```python
from build123d import *

# Parameters (mm, degrees)
SKETCH1_R       = 1
SKETCH1_R_2     = 3.5
SKETCH1_R_3     = 1.5
SKETCH1_W       = 58.004829366
SKETCH1_H       = 74
SKETCH1_W_2     = 12.5
SKETCH1_H_2     = 23.5
EXTRUDE_1_DEPTH = 3


with BuildPart() as part:
    # Sketch1 → Бобышка-Вытянуть1 (new body)
    with BuildSketch(Plane.XY):
        with BuildLine():
            Line((-24.498196466, 18.686253871), (-28.812938034, 21.763271713))
            ThreePointArc((-28.812938034, 21.763271713), (-34.033313652, 22.967935089), (-38.576502294, 20.128397731))
            Line((-38.576502294, 20.128397731), (-42.0602267, 15.24335277))
            ThreePointArc((-42.0602267, 15.24335277), (-43.264890076, 10.022977152), (-40.425352718, 5.47978851))
            Line((-40.425352718, 5.47978851), (-36.440527218, 2.638047245))
            ThreePointArc((-36.440527218, 2.638047245), (-34.281914219, 0.144259766), (-33.504872357, -3.061171876))
            Line((-33.504872357, -3.061171876), (-33.504872357, -48.061171876))
            ThreePointArc((-33.504872357, -48.061171876), (-34.969338451, -51.596705782), (-38.504872357, -53.061171876))
            Line((-38.504872357, -53.061171876), (-42.504872357, -53.061171876))
            ThreePointArc((-42.504872357, -53.061171876), (-47.454619825, -55.111424408), (-49.504872357, -60.061171876))
            Line((-49.504872357, -60.061171876), (-49.500334917, -60.235639257))
            Line((-49.500334917, -60.235639257), (-49.500334917, -66.108369799))
            Line((-49.500334917, -66.108369799), (-49.504872357, -66.28283718))
            ThreePointArc((-49.504872357, -66.28283718), (-47.454619825, -71.232584649), (-42.504872357, -73.28283718))
            Line((-42.504872357, -73.28283718), (-38.504872357, -73.28283718))
            ThreePointArc((-38.504872357, -73.28283718), (-34.969338451, -74.747303275), (-33.504872357, -78.28283718))
            Line((-33.504872357, -78.28283718), (-33.504872357, -123.28283718))
            ThreePointArc((-33.504872357, -123.28283718), (-34.281914219, -126.488268823), (-36.440527218, -128.982056301))
            Line((-36.440527218, -128.982056301), (-40.425352718, -131.823797566))
            ThreePointArc((-40.425352718, -131.823797566), (-43.264890076, -136.366986209), (-42.0602267, -141.587361827))
            Line((-42.0602267, -141.587361827), (-38.576502294, -146.472406787))
            ThreePointArc((-38.576502294, -146.472406787), (-34.033313652, -149.311944145), (-28.812938034, -148.107280769))
            Line((-28.812938034, -148.107280769), (-24.498196466, -145.030262927))
            ThreePointArc((-24.498196466, -145.030262927), (-21.740151192, -143.647892601), (-18.691989124, -143.172004528))
            Line((-18.691989124, -143.172004528), (46.687073776, -143.172004528))
            ThreePointArc((46.687073776, -143.172004528), (49.735235844, -143.647892601), (52.493281118, -145.030262927))
            Line((52.493281118, -145.030262927), (56.808022686, -148.107280769))
            ThreePointArc((56.808022686, -148.107280769), (62.028398304, -149.311944145), (66.571586947, -146.472406787))
            Line((66.571586947, -146.472406787), (70.055311352, -141.587361827))
            ThreePointArc((70.055311352, -141.587361827), (71.259974728, -136.366986209), (68.42043737, -131.823797566))
            Line((68.42043737, -131.823797566), (64.43561187, -128.982056301))
            ThreePointArc((64.43561187, -128.982056301), (62.276998871, -126.488268823), (61.499957009, -123.28283718))
            Line((61.499957009, -123.28283718), (61.499957009, -78.28283718))
            ThreePointArc((61.499957009, -78.28283718), (62.964423103, -74.747303275), (66.499957009, -73.28283718))
            Line((66.499957009, -73.28283718), (70.499957009, -73.28283718))
            ThreePointArc((70.499957009, -73.28283718), (75.449704478, -71.232584649), (77.499957009, -66.28283718))
            Line((77.499957009, -66.28283718), (77.495419569, -66.108369799))
            Line((77.495419569, -66.108369799), (77.495419569, -60.235639257))
            Line((77.495419569, -60.235639257), (77.499957009, -60.061171876))
            ThreePointArc((77.499957009, -60.061171876), (75.449704478, -55.111424407), (70.499957009, -53.061171876))
            Line((70.499957009, -53.061171876), (66.499957009, -53.061171876))
            ThreePointArc((66.499957009, -53.061171876), (62.964423103, -51.596705782), (61.499957009, -48.061171876))
            Line((61.499957009, -48.061171876), (61.499957009, -3.061171876))
            ThreePointArc((61.499957009, -3.061171876), (62.276998871, 0.144259766), (64.43561187, 2.638047245))
            Line((64.43561187, 2.638047245), (68.42043737, 5.47978851))
            ThreePointArc((68.42043737, 5.47978851), (71.259974728, 10.022977152), (70.055311352, 15.24335277))
            Line((70.055311352, 15.24335277), (66.571586947, 20.128397731))
            ThreePointArc((66.571586947, 20.128397731), (62.028398304, 22.967935089), (56.808022686, 21.763271713))
            Line((56.808022686, 21.763271713), (52.493281118, 18.686253871))
            ThreePointArc((52.493281118, 18.686253871), (49.735235844, 17.303883544), (46.687073776, 16.827995472))
            Line((46.687073776, 16.827995472), (-18.691989124, 16.827995472))
            ThreePointArc((-18.691989124, 16.827995472), (-21.740151192, 17.303883544), (-24.498196466, 18.686253871))
        make_face()
        with Locations((-37.997968141, 16.031106158)):
            Circle(SKETCH1_R, mode=Mode.SUBTRACT)
        with Locations((-29.658360325, 17.563764462)):
            Circle(SKETCH1_R, mode=Mode.SUBTRACT)
        with Locations((-36.730320867, 7.647123191)):
            Circle(SKETCH1_R, mode=Mode.SUBTRACT)
        with Locations(Location((-28.390713051, 9.179781495, 0), (0, 0, 180))):
            Circle(SKETCH1_R, mode=Mode.SUBTRACT)
        with Locations((-33.194340596, 12.605443826)):
            Circle(SKETCH1_R_2, mode=Mode.SUBTRACT)
        with Locations(Location((61.189425248, 12.605443826, 0), (0, 0, 180))):
            Circle(SKETCH1_R_2, mode=Mode.SUBTRACT)
        with Locations(Location((56.385797703, 9.179781495, 0), (0, 0, 180))):
            Circle(SKETCH1_R, mode=Mode.SUBTRACT)
        with Locations(Location((64.725405519, 7.647123191, 0), (0, 0, 180))):
            Circle(SKETCH1_R, mode=Mode.SUBTRACT)
        with Locations(Location((57.653444977, 17.563764462, 0), (0, 0, 180))):
            Circle(SKETCH1_R, mode=Mode.SUBTRACT)
        with Locations((65.993052793, 16.031106158)):
            Circle(SKETCH1_R, mode=Mode.SUBTRACT)
        with Locations((65.993052793, -142.375115215)):
            Circle(SKETCH1_R, mode=Mode.SUBTRACT)
        with Locations((57.653444977, -143.907773518)):
            Circle(SKETCH1_R, mode=Mode.SUBTRACT)
        with Locations((64.725405519, -133.991132248)):
            Circle(SKETCH1_R, mode=Mode.SUBTRACT)
        with Locations(Location((56.385797703, -135.523790551, 0), (0, 0, 180))):
            Circle(SKETCH1_R, mode=Mode.SUBTRACT)
        with Locations((61.189425248, -138.949452883)):
            Circle(SKETCH1_R_2, mode=Mode.SUBTRACT)
        with Locations(Location((-33.194340596, -138.949452883, 0), (0, 0, 180))):
            Circle(SKETCH1_R_2, mode=Mode.SUBTRACT)
        with Locations(Location((-28.390713051, -135.523790551, 0), (0, 0, 180))):
            Circle(SKETCH1_R, mode=Mode.SUBTRACT)
        with Locations(Location((-36.730320867, -133.991132248, 0), (0, 0, 180))):
            Circle(SKETCH1_R, mode=Mode.SUBTRACT)
        with Locations(Location((-29.658360325, -143.907773518, 0), (0, 0, 180))):
            Circle(SKETCH1_R, mode=Mode.SUBTRACT)
        with Locations((-37.997968141, -142.375115215)):
            Circle(SKETCH1_R, mode=Mode.SUBTRACT)
        with Locations((55.309957009, -25.561171876)):
            Circle(SKETCH1_R_3, mode=Mode.SUBTRACT)
        with Locations((33.997542326, -136.982004528)):
            Circle(SKETCH1_R_3, mode=Mode.SUBTRACT)
        with Locations((-6.002457674, -136.982004528)):
            Circle(SKETCH1_R_3, mode=Mode.SUBTRACT)
        with Locations(Location((-6.002457674, 10.637995472, 0), (0, 0, 180))):
            Circle(SKETCH1_R_3, mode=Mode.SUBTRACT)
        with Locations(Location((33.997542326, 10.637995472, 0), (0, 0, 180))):
            Circle(SKETCH1_R_3, mode=Mode.SUBTRACT)
        with Locations((13.997542326, -132.673899794)):
            Circle(SKETCH1_R, mode=Mode.SUBTRACT)
        with Locations(Location((13.997542326, -105.173899794, 0), (0, 0, 180))):
            Circle(SKETCH1_R, mode=Mode.SUBTRACT)
        with Locations((-27.314872357, -25.561171876)):
            Circle(SKETCH1_R_3, mode=Mode.SUBTRACT)
        with Locations((55.309957009, -100.78283718)):
            Circle(SKETCH1_R_3, mode=Mode.SUBTRACT)
        with Locations((-27.314872357, -100.78283718)):
            Circle(SKETCH1_R_3, mode=Mode.SUBTRACT)
        with Locations((-40.750334917, -63.172004528)):
            Circle(SKETCH1_R_2, mode=Mode.SUBTRACT)
        with Locations((-46.650334917, -63.172004528)):
            Circle(SKETCH1_R, mode=Mode.SUBTRACT)
        with Locations(Location((-34.850334917, -63.172004528, 0), (0, 0, 180))):
            Circle(SKETCH1_R, mode=Mode.SUBTRACT)
        with Locations((-40.487335358, -69.256322997)):
            Circle(SKETCH1_R, mode=Mode.SUBTRACT)
        with Locations(Location((-40.487335358, -57.087686059, 0), (0, 0, 180))):
            Circle(SKETCH1_R, mode=Mode.SUBTRACT)
        with Locations((68.48242001, -57.087686059)):
            Circle(SKETCH1_R, mode=Mode.SUBTRACT)
        with Locations(Location((68.48242001, -69.256322997, 0), (0, 0, 180))):
            Circle(SKETCH1_R, mode=Mode.SUBTRACT)
        with Locations((62.845419569, -63.172004528)):
            Circle(SKETCH1_R, mode=Mode.SUBTRACT)
        with Locations(Location((74.645419569, -63.172004528, 0), (0, 0, 180))):
            Circle(SKETCH1_R, mode=Mode.SUBTRACT)
        with Locations(Location((68.745419569, -63.172004528, 0), (0, 0, 180))):
            Circle(SKETCH1_R_2, mode=Mode.SUBTRACT)
        with Locations((13.997542326, -38.172004528)):
            Rectangle(SKETCH1_W, SKETCH1_H, mode=Mode.SUBTRACT)
        with Locations((13.997542326, -118.923899794)):
            Rectangle(SKETCH1_W_2, SKETCH1_H_2, mode=Mode.SUBTRACT)
        with BuildLine():
            Line((32.005035086, -106.680183908), (43.167511474, -114.653381328))
            ThreePointArc((43.167511474, -114.653381328), (44.206331249, -114.728815499), (44.748749668, -113.839647857))
            Line((44.748749668, -113.839647857), (44.748749668, -100.78283718))
            Line((44.748749668, -100.78283718), (44.748749668, -97.326690866))
            ThreePointArc((44.748749668, -97.326690866), (44.416252596, -95.953946124), (43.492464249, -94.885490453))
            Line((43.492464249, -94.885490453), (32.329987861, -86.912293033))
            ThreePointArc((32.329987861, -86.912293033), (31.291168087, -86.836858862), (30.748749668, -87.726026504))
            Line((30.748749668, -87.726026504), (30.748749668, -100.78283718))
            Line((30.748749668, -100.78283718), (30.748749668, -104.238983495))
            ThreePointArc((30.748749668, -104.238983495), (31.081246739, -105.611728237), (32.005035086, -106.680183908))
        make_face(mode=Mode.SUBTRACT)
        with BuildLine():
            Line((-2.753665015, -100.78283718), (-2.753665015, -87.726026504))
            ThreePointArc((-2.753665015, -87.726026504), (-3.296083435, -86.836858862), (-4.334903209, -86.912293033))
            Line((-4.334903209, -86.912293033), (-15.497379597, -94.885490453))
            ThreePointArc((-15.497379597, -94.885490453), (-16.421167944, -95.953946124), (-16.753665015, -97.326690866))
            Line((-16.753665015, -97.326690866), (-16.753665015, -100.78283718))
            Line((-16.753665015, -100.78283718), (-16.753665015, -113.839647857))
            ThreePointArc((-16.753665015, -113.839647857), (-16.211246596, -114.728815499), (-15.172426822, -114.653381328))
            Line((-15.172426822, -114.653381328), (-4.009950434, -106.680183908))
            ThreePointArc((-4.009950434, -106.680183908), (-3.086162087, -105.611728237), (-2.753665015, -104.238983495))
            Line((-2.753665015, -104.238983495), (-2.753665015, -100.78283718))
        make_face(mode=Mode.SUBTRACT)
    extrude(amount=-EXTRUDE_1_DEPTH)


solid = part.part
```
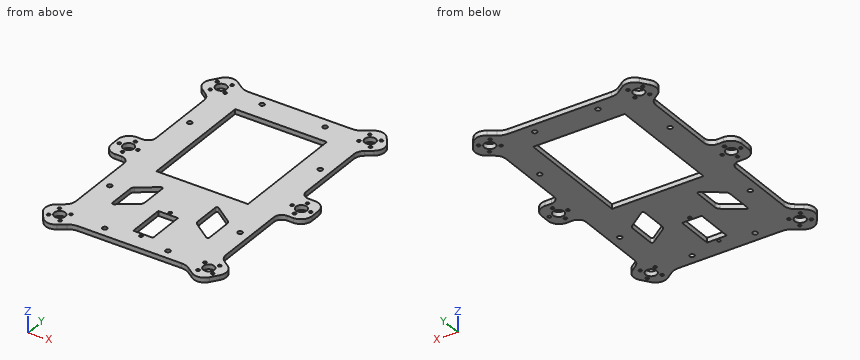
CAD build for the part. Positions are in the model's coordinates, mm. Round coordinates to 2 decimals unless told otherwise and drop trailing zeros. Loops run counter-clockwise (first coordinate to the right, second up) from the corner with the lowest first, then second, coordinate; pieces in that order, holes last. Notation, with made-up numbers: M 81,-33.75 L 94,-33.75 A24 cw 94,-4.75 Z; hole C 31.25,41 d4. An arc over 180 degrees is marked long. Return JSON: item names as keys, results as strings. Group by question number.
(1) Wall check: probe 1 along X at (y, z) = (-103.5, -1.05); probe 2 along Y at (x, z) = (23, -2.4); probe 3 along Y at (x, z) = (14.5, -2.35). Give the ranges that are in metal, low to high. Write a range as [from, to].
(2) Saw through at D-D, the plane z = -1.85. Give the number of separate pieces and of enclosed holes in the cut face, and give its area (3 significant figures).
(3) Saw through at B-B, the plane y = -38. List the corners of the cut face in (x, z), and give its area (3 significant figures).
(4) Saw through at C-C, the plane y = -125. List the corners of the cut face in (x, z).
(5) Drop flat-ended pins along their axis: P1, Ø5.5, axis at x = -33.19, y = 12.61, coming from the -Z side; P2, Ø3, axis at x = 62.85, y = -63.17, coming from the -Z side; P3, Ø0.9, axis at x = 68.5, z = -1.5, coming from the -Y side; P4, Ø1.5, axis at x = -40, z = -1, coming from the +Y side. Give the stop position or say it passes through.
(6) Saw through at A-A, the plane x = 17. List the corners of the cut face in (y, z), and give its area (4 significant figures).
Answer list:
{
 "1": {"probe 1": "[-33.5, -16.75], [-2.75, 30.75], [44.75, 61.5]", "probe 2": "[-143.17, -75.17], [-1.17, 16.83]", "probe 3": "[-143.17, -133.54], [-131.81, -130.67], [-107.17, -106.04], [-104.31, -75.17], [-1.17, 16.83]"},
 "2": {"separate pieces": "1", "enclosed holes": "44", "area": "11,100 mm2"},
 "3": {"outline": "M -33.5,-3 L -15,-3 L -15,0 L -33.5,0 Z; M 43,-3 L 61.5,-3 L 61.5,0 L 43,0 Z", "area": "111 mm2"},
 "4": {"outline": "M -33.72,-3 L 7.75,-3 L 7.75,0 L -33.72,0 Z; M 20.25,-3 L 61.71,-3 L 61.71,0 L 20.25,0 Z"},
 "5": {"P1": "through", "P2": "z = -3", "P3": "y = -144.4", "P4": "y = 19.18"},
 "6": {"outline": "M -143.17,-3 L -130.67,-3 L -130.67,0 L -143.17,0 Z; M -107.17,-3 L -75.17,-3 L -75.17,0 L -107.17,0 Z; M -1.17,-3 L 16.83,-3 L 16.83,0 L -1.17,0 Z", "area": "187.5 mm2"}
}
